from build123d import *

# Parameters (mm, degrees)
ESQUISSE1_R        = 2
BOSS_EXTRU_1_DEPTH = 128.4


with BuildPart() as part:
    # Esquisse1 → Boss.-Extru.1 (new, symmetric)
    with BuildSketch(Plane.XY):
        Circle(ESQUISSE1_R)
    extrude(amount=BOSS_EXTRU_1_DEPTH, both=True)

    # Esquisse2 → Enlèvement de matière-Révolution1 (revolve, cut)
    with BuildSketch(Plane(origin=(0, 0, 0), x_dir=(1, 0, 0), z_dir=(0, 1, 0))):
        with BuildLine():
            Line((6.35, 128.4), (-6.35, 128.4))
            ThreePointArc((-6.35, 128.4), (-1.17e-15, 122.05000000000001), (6.35, 128.4))
        make_face()
    enl_vement_de_mati_re_r_volution1 = revolve(axis=Axis((6.35, 0, -128.4), (-1, 0, 0)), mode=Mode.SUBTRACT)

    # Symétrie1: Enlèvement de matière-Révolution1 across plane
    add(enl_vement_de_mati_re_r_volution1.mirror(Plane.XY), mode=Mode.SUBTRACT)


solid = part.part
Can you work these out from the model? Positions are in its coordinate system, mm. Coordinates: 2 decimals unless noted, no trailing zeros. Write each loop counter-clockwise with the first axis right and the second up, starting at its lowest first coordinate (ties: lowest second). Pieces come first, ordered by that corner, then holes. Notation, with made-up numbers: (18, 11.25) -> (55, 11.25) arc R17 cw to (55, 25.25) -> close; hole circle Ø7 at (-5.5, 49). An arc over 180 degrees is marked (long way). Write each question's results on one line, items separated by ' | '. Start each with the question number.
Q1. Imagine slicing it at C-C (x = 1.35). Write out the boundary of the cut face in (y, z).
Q2. Imagine slicing it at A-A (y = -1.2). Write out the boundary of the cut face in (x, z), then the cut area to 3 significant figures.
Q3. Imagine slicing it at B-B (z = 87). Write out the boundary of the cut face in (x, y).
Q4. I'm going to push flat-ended pins straight in: pin 1 (1.5 mm diameter, centred on x = 0.5, y = -0.5, fed in from -Z); pin 2 (1 mm diameter, centred on x = -1, y = 0.5, fed in from -Z); pin 3 (2 mm diameter, centred on y = -1, z = -42.5, fed in from +X). Where does each tip first touch, or does it pass through?
Q5. If I drill on probe 1 along Y at (x, z) = (-0.4, -36); probe 2 along Z at (x, y) = (0.7, 0.3); probe 3 along Z at (x, y) = (1.85, 0.3), over which ranges is the centre line in solid material (lowest first)?
Taken from the geometry:
1) outline: (-1.48, -122.37) arc R6.2 cw to (1.48, -122.37) -> (1.48, 122.37) arc R6.2 cw to (-1.48, 122.37) -> close
2) outline: (-1.6, -122.37) arc R6.24 cw to (1.6, -122.37) -> (1.6, 122.37) arc R6.24 cw to (-1.6, 122.37) -> close | area: 782 mm^2
3) outline: circle Ø4 at (0, 0)
4) pin 1: stops at z = -122.22 | pin 2: stops at z = -122.26 | pin 3: stops at x = 2
5) probe 1: y = -1.96 to 1.96 | probe 2: z = -122.1 to 122.1 | probe 3: z = -122.33 to 122.33
